Here's how the part is built. I have some questions about the finished solid (model axes, mm). Round coordinates to 2 decimals unless told otherwise and drop trailing zeros. Write each loop counter-clockwise with the first axis right and the second up, starting at its lowest first coordinate (ties: lowest second). Pieces come first, ordered by that corner, then holes. Notation, with made-up numbers: M -37,-39 L 6,-39 A24 cw 6,-6 Z; hole C -22,-17.75 d11. An arc over 180 degrees is marked long. Use a Markdown table: item, result. Add a question column.
Autodesk Inventor part; units mm, degrees
ref_plane "YZ Plane" through (0, 0, 0) normal (1, 0, 0) x (0, 1, 0)
ref_plane "XZ Plane" through (0, 0, 0) normal (0, 1, 0) x (-1, 0, 0)
ref_plane "XY Plane" through (0, 0, 0) normal (0, 0, 1) x (1, 0, 0)
sketch "Sketch1" plane through (0, 0, 0) normal (0, 0, 1) x (1, 0, 0)
  arc A0 (0, -9.7409) -> (0, 9.7409) centre (0, 0) ccw
  arc A1 (-172.72, 9.7409) -> (-172.72, -9.7409) centre (-172.72, 0) ccw
  line L0 (-172.72, 9.7409) -> (0, 9.7409)
  line L1 (0, -9.7409) -> (-172.72, -9.7409)
  circle A2 centre (-172.72, 0) radius 3.2512
  circle A3 centre (0, 0) radius 3.2512
  circle A4 centre (-83.82, 0) radius 3.2512
  dimension "d0" = 19.4818
  dimension "d1" = 19.4818
  dimension "d2" = 172.72
  dimension "d3" = 6.5024
  dimension "d4" = 6.5024
  dimension "d12" = 6.5024
  dimension "d13" = 9.7409
  dimension "d14" = 88.9
extrude "Extrusion1" add sketch "Sketch1" along normal blind 2.54 contours L1 A1 L0 A0 | A4
sketch "Sketch2" plane through (0, 0, 0) normal (0, 0, -1) x (-1, 0, 0)
  circle A0 centre (99.06, 0) radius 3.175
  circle A1 centre (172.72, 0) radius 3.2512
  circle A2 centre (0, 0) radius 3.2512
  line L0 (172.72, 9.7409) -> (0, 9.7409)
  arc A3 (0, 9.7409) -> (0, -9.7409) centre (0, 0) ccw
  line L1 (0, -9.7409) -> (172.72, -9.7409)
  arc A4 (172.72, -9.7409) -> (172.72, 9.7409) centre (172.72, 0) ccw
  point P0 (86.36, 9.7409)
  dimension "d7" = 6.35
  dimension "d11" = 73.66
extrude "Extrusion2" cut sketch "Sketch2" against normal through all contours A0
equation "\"d0\" = d1"
properties part number "ArmConnector2"
Item 1: If we mould it in two halves opening along Y, with no side actions, what happens to faces 1 (the face through (9.74, 0.21, 1.25)), 2 (the face through (-0.423, -3.224, 1.252)), 3 (the face through (-88, 0, 2.54))? For each: +Y half, -Y half, draft (parallel to the pull), parting line (faces both ways), or undercut.
Item 2: I need wall thicknesses on probe 1 along X at (y, z) = (-0.5, 1.7); probe 2 along Y at (x, z) = (-172.72, 1.4); probe 3 along X at (y, z) = (-1.75, 1.05). Which ranges of each line are inside material? Lowest first, please. Write a range as from..to.
Item 3: Imagine slicing it at D-D on y = 6. List the corners of the cut face in (x, z) for me.
Item 4: For pin 1 Ø6 at (x, y) = (-172.72, 0) entering from +Z; pin 2 Ø1.5 at (y, z) = (-6, 1.5) entering from +X; pin 3 Ø1.5 at (y, z) = (5.5, 1) entering from +X; pin 4 Ø1.5 at (y, z) = (1, 0.5) entering from +X, each with a flat end and sliding along its axis, tell me the tip position at first contact or that it passes through.
Item 5: Imagine slicing it at B-B on z = 0.4. List the corners of the cut face in (x, y) for me (3 decimals), plus the area to 3 significant figures.
Item 6: Imagine slicing it at C-C on y = -5.5. List the corners of the cut face in (x, z) for me, plus the area to 3 significant figures.
Item 7: Imagine slicing it at A-A on x = -99.06. List the corners of the cut face in (y, z) for me (3 decimals), plus the area to 3 significant figures.
The answers:
| question | item | result |
|---|---|---|
| 1 | face 1 | parting line |
| 1 | face 2 | undercut |
| 1 | face 3 | draft |
| 2 | probe 1 | -182.45..-175.93, -169.51..-102.2, -95.92..-3.21, 3.21..9.73 |
| 2 | probe 2 | -9.74..-3.25, 3.25..9.74 |
| 2 | probe 3 | -182.3..-175.46, -169.98..-101.71, -96.41..-2.74, 2.74..9.58 |
| 3 | outline | M -180.39,0 L 7.67,0 L 7.67,2.54 L -180.39,2.54 Z |
| 4 | pin 1 | through |
| 4 | pin 2 | x = 8.21 |
| 4 | pin 3 | x = 8.5 |
| 4 | pin 4 | x = 9.74 |
| 5 | outline | M -172.72,-9.741 L 0,-9.741 A9.741 ccw 0,9.741 L -172.72,9.741 A9.741 ccw Z; hole C -172.72,0 d6.502; hole C -99.06,0 d6.35; hole C 0,0 d6.502 |
| 5 | area | 3,560 mm² |
| 6 | outline | M -180.76,0 L 8.04,0 L 8.04,2.54 L -180.76,2.54 Z |
| 6 | area | 480 mm² |
| 7 | outline | M -9.741,0 L -3.175,0 L -3.175,2.54 L -9.741,2.54 Z; M 3.175,0 L 9.741,0 L 9.741,2.54 L 3.175,2.54 Z |
| 7 | area | 33.4 mm² |
